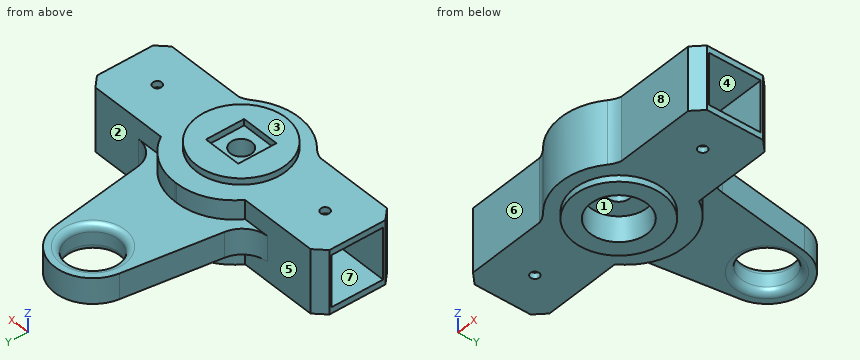
```python
from build123d import *

# Parameters (mm, degrees)
CROQUIS1_R                   = 15
CROQUIS1_R_2                 = 10
SALIENTE_EXTRUIR1_DEPTH      = 12.5
CORTAR_EXTRUIR2_DEPTH        = 78.778499901
CORTAR_EXTRUIR2_DEPTH_BACK   = 78.778499901
CROQUIS3_W                   = 7.5
CROQUIS3_H                   = 47.5
REDONDEO3_R                  = 22.5
CROQUIS4_W                   = 35
CROQUIS4_H                   = 30
CROQUIS4_R                   = 1.75
SALIENTE_EXTRUIR2_DEPTH      = 25
CROQUIS5_W                   = 20.2
CROQUIS5_H                   = 20.2
CORTAR_EXTRUIR3_DEPTH        = 30
REDONDEO4_R                  = 10
CHAFL_N1_SIZE                = 4
REDONDEO6_R                  = 2.5
SALIENTE_EXTRUIR3_DEPTH      = 2.5
SALIENTE_EXTRUIR3_DEPTH_BACK = 27.5
CROQUIS6_R                   = 17.5
CROQUIS6_R_2                 = 11.1
CROQUIS8_R                   = 17.5
CROQUIS8_R_2                 = 4.2
SALIENTE_EXTRUIR4_DEPTH      = 20
CORTAR_EXTRUIR4_DEPTH        = 96.753237788
CORTAR_EXTRUIR4_DEPTH_BACK   = 2.5
CROQUIS9_W                   = 15
CROQUIS9_H                   = 15
CROQUIS9_R                   = 4.2


with BuildPart() as part:
    # Croquis1 → Saliente-Extruir1 (new, symmetric)
    with BuildSketch(Plane.XY):
        with BuildLine():
            Line((-23.009443154, 3.997898972), (-14.844802035, 60.31420332))
            ThreePointArc((-14.844802035, 60.31420332), (0, 73.162029407), (14.844802035, 60.31420332))
            Line((14.844802035, 60.31420332), (23.009443154, 3.997898972))
            ThreePointArc((23.009443154, 3.997898972), (0, -22.587970593), (-23.009443154, 3.997898972))
        make_face()
        Circle(CROQUIS1_R, mode=Mode.SUBTRACT)
        with Locations((0, 58.162029407)):
            Circle(CROQUIS1_R_2, mode=Mode.SUBTRACT)
    extrude(amount=SALIENTE_EXTRUIR1_DEPTH, both=True)

    # Croquis3 → Cortar-Extruir2 (cut, two sides: drawn at the far end of the back side and taken through both)
    with BuildSketch(Plane(origin=(0, 0, 0), x_dir=(0, 0, -1), z_dir=(1, 0, 0)).offset(-CORTAR_EXTRUIR2_DEPTH_BACK)):
        with Locations((8.75, 49.412029407)):
            Rectangle(CROQUIS3_W, CROQUIS3_H)
        with Locations((-8.75, 49.412029407)):
            Rectangle(CROQUIS3_W, CROQUIS3_H)
    extrude(amount=CORTAR_EXTRUIR2_DEPTH + CORTAR_EXTRUIR2_DEPTH_BACK, mode=Mode.SUBTRACT)

    # Redondeo3
    redondeo3_edges = [part.edges().sort_by_distance(p)[0] for p in [
        (-19.868614717, 25.662029407, 8.75),
        (-19.868614717, 25.662029407, -8.75),
        (19.868614717, 25.662029407, -8.75),
        (19.868614717, 25.662029407, 8.75),
    ]]
    fillet(redondeo3_edges, radius=REDONDEO3_R)

    # Croquis4 → Saliente-Extruir2 (add)
    # profile 1 of 2: a face of its own
    with BuildSketch(Plane(origin=(0, 0, -12.5), x_dir=(-1, 0, 0), z_dir=(0, 0, -1))):
        with Locations((-36.5, 0)):
            Rectangle(CROQUIS4_W, CROQUIS4_H)
        with Locations((-39, 0)):
            Circle(CROQUIS4_R, mode=Mode.SUBTRACT)
    # profile 2 of 2: a face of its own
    with BuildSketch(Plane(origin=(0, 0, -12.5), x_dir=(-1, 0, 0), z_dir=(0, 0, -1))):
        with Locations((36.5, 0)):
            Rectangle(CROQUIS4_W, CROQUIS4_H)
        with Locations(Location((39, 0, 0), (0, 0, 180))):
            Circle(CROQUIS4_R, mode=Mode.SUBTRACT)
    extrude(amount=-SALIENTE_EXTRUIR2_DEPTH)

    # Croquis5 → Cortar-Extruir3 (cut)
    with BuildSketch(Plane(origin=(54, 0, 0), x_dir=(0, 0, -1), z_dir=(1, 0, 0))):
        Rectangle(CROQUIS5_W, CROQUIS5_H)
    cortar_extruir3 = extrude(amount=-CORTAR_EXTRUIR3_DEPTH, mode=Mode.SUBTRACT)

    # Simetría1: Cortar-Extruir3 across plane
    add(cortar_extruir3.mirror(Plane(origin=(0, 0, 0), x_dir=(0, 0, 1), z_dir=(1, 0, 0))), mode=Mode.SUBTRACT)

    # Redondeo4
    # the kernel refuses this fillet: 10 mm, written as the material it adds along each edge
    with BuildSketch(Plane(origin=(-19, -12.738063876, -12.5), x_dir=(0.674519649650932, -0.7382568944715545, 0), z_dir=(0, 0, 1))) as redondeo4_piece_1:
        with BuildLine():
            CenterArc((7.103598198, -9.920648267), REDONDEO4_R, 97.222764243, 25.690637502)
            Line((1.669889938, -1.525720362), (0, 0))
            ThreePointArc((0, 0), (2.92316209, -0.184492778), (5.846324181, 0))
        make_face()
    extrude(amount=25)
    with BuildSketch(Plane(origin=(19, -12.738063876, -12.5), x_dir=(0, -1, 0), z_dir=(0, 0, 1))) as redondeo4_piece_2:
        with BuildLine():
            CenterArc((11.935952539, 2.532470413), REDONDEO4_R, 194.669738911, 25.690637502)
            ThreePointArc((4.316089134, -3.943460538), (2.282488571, -1.835527204), (0, 0))
            Line((0, 0), (2.261936124, 0))
        make_face()
    extrude(amount=25)
    with BuildSketch(Plane(origin=(21.414377435, 15, -5), x_dir=(1, 0, 0), z_dir=(0, 0, 1)), Plane(origin=(-21.414377435, 15, 5), x_dir=(-1, 0, 0), z_dir=(0, 0, -1))) as redondeo4_piece_3:
        with BuildLine():
            CenterArc((REDONDEO4_R * 0.865476417736, REDONDEO4_R), REDONDEO4_R, 188.249168565, 81.750831435)
            Line((-REDONDEO4_R * 0.12417705124, REDONDEO4_R * 0.85652173913), (0, 0))
            Line((0, 0), (REDONDEO4_R * 0.865476417736, 0))
        make_face()
    extrude(amount=10)

    # Chaflán1
    chafl_n1_edges = [part.edges().sort_by_distance(p)[0] for p in [
        (-54, 15, 0),
        (-54, -15, 0),
        (54, -15, 0),
        (54, 15, 0),
    ]]
    chamfer(chafl_n1_edges, length=CHAFL_N1_SIZE)

    # Redondeo6
    redondeo6_edges = [part.edges().sort_by_distance(p)[0] for p in [
        (-10, 58.162029407, -5),
        (-10, 58.162029407, 5),
    ]]
    fillet(redondeo6_edges, radius=REDONDEO6_R)

    # Croquis6 → Saliente-Extruir3 (add, two sides: drawn at the far end of the back side and taken through both)
    with BuildSketch(Plane.XY.offset(12.5).offset(-SALIENTE_EXTRUIR3_DEPTH_BACK)):
        Circle(CROQUIS6_R)
        Circle(CROQUIS6_R_2, mode=Mode.SUBTRACT)
    extrude(amount=SALIENTE_EXTRUIR3_DEPTH + SALIENTE_EXTRUIR3_DEPTH_BACK)

    # Croquis8 → Saliente-Extruir4 (add)
    with BuildSketch(Plane.XY.offset(15)):
        Circle(CROQUIS8_R)
        Circle(CROQUIS8_R_2, mode=Mode.SUBTRACT)
    extrude(amount=-SALIENTE_EXTRUIR4_DEPTH)

    # Croquis9 → Cortar-Extruir4 (cut, two sides: drawn at the far end of the back side and taken through both)
    with BuildSketch(Plane.XY.offset(15).offset(-CORTAR_EXTRUIR4_DEPTH_BACK)):
        Rectangle(CROQUIS9_W, CROQUIS9_H)
        Circle(CROQUIS9_R, mode=Mode.SUBTRACT)
    extrude(amount=CORTAR_EXTRUIR4_DEPTH + CORTAR_EXTRUIR4_DEPTH_BACK, mode=Mode.SUBTRACT)


solid = part.part
```
Could you check a few things on this model? Use its own coordinates, in mm. Face numbers are marked on the shaded views. A direction names the side the tool comes from. Round coordinates to 2 decimals unless told otherwise and drop trailing zeros. Write each loop counter-clockwise with the first axis right and the second up, starting at its lowest first coordinate (ties: lowest second). Pieces come first, ordered by that corner, then holes. Notation, with made-up numbers: M 89,-18.5 L 136,-18.5 A25 cw 136,16.5 Z; hole C 75.5,-13 d3. An arc over 180 degrees is marked long. Write each question's results on one line, items separated by ' | '. Start each with the question number.
1. I need wall thicknesses on L1, parallel to X at y = 0, z = -9.75; L2, parallel to Y at x = 37.5, z = 8; L3, parallel to Y at x = 39, z = -11.5. Which ranges of each line are inside material? Lowest first, please. Write a range as from..to.
2. Imagine slicing it at A-A on x = -39. List the corners of the cut face in (y, z) for me.
3. Imagine slicing it at D-D on y = 21. List the corners of the cut face in (x, z) for me.
4. Imagine slicing it at B-B on x = 42. List the corners of the cut face in (y, z) for me.
5. Thinking about a two-plate mould opening in Y: for the marked faces 1, 2 and 3, which applies, +Y half, -Y half, draft (parallel to the pull), parting line (faces both ways), or undercut?
6. Imagine slicing it at C-C on y = 0. Count the separate pieces of the cut face and the enclosed holes in it, and give its area (3 significant figures).
7. I'm going to push flat-ended pins straight in: pin 1 Ø10 at (x, z) = (37, 2) entering from +Y; pin 2 Ø16 at (x, y) = (32.5, -1) entering from -Z; pin 3 Ø2 at (x, z) = (-37.5, 7.5) entering from -Y. Where does each tip first touch, or does it pass through?
8. On a 3-axis mill with a long thin cutter (end or side, diameter ignored), from which of +Z, -Z, +X, -X, +Y, -Y can I reach the whole of each face in a straight line? I mean the marked faces 4, 5, 6, 7 and 8. Say none if no direction works.
Result sheet:
1) L1: x = -24..-11.1, 11.1..24 | L2: y = -15..-10.1, 10.1..15 | L3: y = -15..-1.75, 1.75..15
2) outline: M -15,-12.5 L -1.75,-12.5 L -1.75,-10.1 L -10.1,-10.1 L -10.1,10.1 L -1.75,10.1 L -1.75,12.5 L -15,12.5 Z; M 1.75,-12.5 L 15,-12.5 L 15,12.5 L 1.75,12.5 L 1.75,10.1 L 10.1,10.1 L 10.1,-10.1 L 1.75,-10.1 Z
3) outline: M -20.9,-5 L -14.11,-5 L -14.11,-12.5 L 14.11,-12.5 L 14.11,-5 L 20.9,-5 L 20.9,5 L 14.11,5 L 14.11,12.5 L -14.11,12.5 L -14.11,5 L -20.9,5 Z
4) outline: M -15,-12.5 L 15,-12.5 L 15,12.5 L -15,12.5 Z; hole M -10.1,-10.1 L 10.1,-10.1 L 10.1,10.1 L -10.1,10.1 Z
5) face 1: undercut | face 2: +Y half | face 3: draft
6) separate pieces: 6 | enclosed holes: 0 | area: 1,220 mm^2
7) pin 1: stops at y = 15 | pin 2: stops at z = -12.5 | pin 3: stops at y = -15
8) face 4: +X | face 5: -X, +Y | face 6: +Z, -Z, -X, -Y | face 7: -X | face 8: +Z, -Z, +X, -Y
